Source: CAD feature listing. Evaluate the final solid. Frame: model axes, mm. Face numbers are marked on the shaded views. A direction names the side the tool comes from. Round coordinates to 2 decimals unless told otherwise and drop trailing zeros. Order: outer loops, then holes, each group sorted by start corner. A loop starts at its lowest first (then second) coordinate and runs counter-clockwise, first axis right, second up. Notation, with made-up numbers: (85.5, 7.25) -> (101.5, 7.25) arc R24 cw to (101.5, 25.25) -> close; hole circle Ø9 at (59.25, -34.75). An arc over 180 degrees is marked (long way). Answer as CSV lines item,"result".
from build123d import *

# Parameters (mm, degrees)
F0_W      = 165.1
F0_H      = 44.45
F1_DEPTH  = 22.86
F2_R      = 5.08
F3_DEPTH  = 5.334
F4_R      = 2.794
F5_DEPTH  = 25.4
F6_W      = 9.398
F6_H      = 16.51
F7_DEPTH  = 21.59
F8_W      = 2.286
F8_H      = 16.51
F9_DEPTH  = 8.128
F11_DEPTH = 25.4
F12_R     = 1.27
F13_DEPTH = 6.35


with BuildPart() as f1:
    # F0 (on Front) → F1 (new body)
    with BuildSketch(Plane.XZ):
        with Locations((22.303157, 29.753123)):
            Rectangle(F0_W, F0_H)
    extrude(amount=F1_DEPTH)

    # F2 (on face) → F3 (join)
    with BuildSketch(Plane(origin=(-60.246843, 0, 0), x_dir=(0, -1, 0), z_dir=(-1, 0, 0))):
        with Locations((9.652, 36.103123)):
            Circle(F2_R)
    extrude(amount=F3_DEPTH)

    # F4 (on face) → F5 (join)
    with BuildSketch(Plane(origin=(-65.580843, 0, 0), x_dir=(0, -1, 0), z_dir=(-1, 0, 0))):
        with Locations((9.652, 36.103123)):
            Circle(F4_R)
    extrude(amount=F5_DEPTH)

    # F6 (on face) → F7 (join)
    with BuildSketch(Plane.XZ.offset(22.86)):
        with Locations((-36.497843, 39.913123)):
            Rectangle(F6_W, F6_H)
        with Locations((-15.542843, 39.913123)):
            Rectangle(F6_W, F6_H)
        with Locations((5.412157, 39.913123)):
            Rectangle(F6_W, F6_H)
        with Locations((26.367157, 39.913123)):
            Rectangle(F6_W, F6_H)
        with Locations((47.322157, 39.913123)):
            Rectangle(F6_W, F6_H)
        with Locations((68.277157, 39.913123)):
            Rectangle(F6_W, F6_H)
        with Locations((89.232157, 39.913123)):
            Rectangle(F6_W, F6_H)
    extrude(amount=F7_DEPTH)

    # F8 (on face) → F9 (join)
    with BuildSketch(Plane.YZ.offset(104.853157)):
        with Locations((-1.143, 29.753123)):
            Rectangle(F8_W, F8_H)
    extrude(amount=F9_DEPTH)

    # F10 (on face) → F11 (cut)
    with BuildSketch(Plane.XZ.offset(2.286)):
        with BuildLine():
            Line((112.981157, 38.008123), (104.853157, 38.008123))
            Line((104.853157, 38.008123), (111.457157, 33.055123))
            ThreePointArc((111.457157, 33.055123), (112.578924, 31.711006), (112.981157, 30.007123))
            Line((112.981157, 30.007123), (112.981157, 31.912123))
            Line((112.981157, 31.912123), (112.981157, 38.008123))
        make_face()
        with BuildLine():
            Line((112.981157, 27.594123), (112.981157, 29.499123))
            ThreePointArc((112.981157, 29.499123), (112.578924, 27.795239), (111.457157, 26.451123))
            Line((111.457157, 26.451123), (104.853157, 21.498123))
            Line((104.853157, 21.498123), (112.981157, 21.498123))
            Line((112.981157, 21.498123), (112.981157, 27.594123))
        make_face()
        with BuildLine():
            Line((110.339557, 32.039123), (106.072357, 35.239523))
            ThreePointArc((106.072357, 35.239523), (105.27438, 35.311476), (104.853157, 34.629923))
            Line((104.853157, 34.629923), (104.853157, 29.753123))
            Line((104.853157, 29.753123), (111.355557, 29.753123))
            Line((111.355557, 29.753123), (111.355557, 30.007123))
            ThreePointArc((111.355557, 30.007123), (111.087402, 31.143045), (110.339557, 32.039123))
        make_face()
        with BuildLine():
            Line((111.355557, 29.753123), (104.853157, 29.753123))
            Line((104.853157, 29.753123), (104.853157, 24.876323))
            ThreePointArc((104.853157, 24.876323), (105.27438, 24.194769), (106.072357, 24.266723))
            Line((106.072357, 24.266723), (110.339557, 27.467123))
            ThreePointArc((110.339557, 27.467123), (111.087402, 28.3632), (111.355557, 29.499123))
            Line((111.355557, 29.499123), (111.355557, 29.753123))
        make_face()
    extrude(amount=-F11_DEPTH, mode=Mode.SUBTRACT)

    # F12 (on face) → F13 (cut)
    with BuildSketch(Plane(origin=(0, 0, 0), x_dir=(-1, 0, 0), z_dir=(0, 1, 0))):
        with Locations((47.546843, 29.753123)):
            Circle(F12_R)
    extrude(amount=-F13_DEPTH, mode=Mode.SUBTRACT)


solid = f1.part
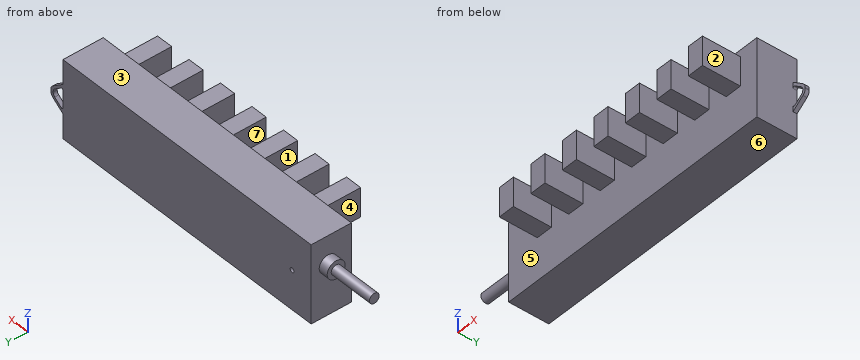
1. Section query A-A on y = -27.5. Return loops of the section in (x, z), and give its area (3 significant figures).
Results below:
outline,"(-41.2, 31.66) -> (-31.8, 31.66) -> (-31.8, 48.17) -> (-41.2, 48.17) -> close; (-20.24, 31.66) -> (-10.84, 31.66) -> (-10.84, 48.17) -> (-20.24, 48.17) -> close; (0.71, 31.66) -> (10.11, 31.66) -> (10.11, 48.17) -> (0.71, 48.17) -> close; (21.67, 31.66) -> (31.07, 31.66) -> (31.07, 48.17) -> (21.67, 48.17) -> close; (42.62, 31.66) -> (52.02, 31.66) -> (52.02, 48.17) -> (42.62, 48.17) -> close; (63.58, 31.66) -> (72.98, 31.66) -> (72.98, 48.17) -> (63.58, 48.17) -> close; (84.53, 31.66) -> (93.93, 31.66) -> (93.93, 48.17) -> (84.53, 48.17) -> close"
area,"1,090 mm2"
2. Line query: L1, parallel to Y at x = 18.5, z = 33.5; L2, parallel to X at y = -22.5, z = 36.5; L3, parallel to Z at x = -11.5, y = -26. Output: solid intervals per line, ascending. Write a range as [from, to].
Results below:
L1,"[-22.86, 0]"
L2,"[-60.25, 104.85]"
L3,"[31.66, 48.17]"
3. Reachability of the marked faces 1, 2 and 3 from +Z, -Z, +X, -X, +Y, -Y: full face, straight path, thin tool, end or side. Return the list, or none.
Results below:
face 1,"+Z, -Z, -Y"
face 2,"+Z, -Z, +X, -Y"
face 3,"+Z, +X, -X, +Y, -Y"
4. Pin query (flat end, axial travel): pin 1 (18 mm diameter, centred on y = -31.5, z = 41.5, fed in from -X); pin 2 (8.5 mm diameter, centred on y = -38, z = 40, fed in from -X); pin 3 (10.5 mm diameter, centred on x = 91, y = -35.5, fed in from +Z). Return the tip coordinate at first contact, or that it passes through.
Results below:
pin 1,"x = -60.25"
pin 2,"x = -41.2"
pin 3,"z = 48.17"
5. Section query C-C on z = 19. Return loops of the section in (x, y).
Results below:
outline,"(-60.25, -22.86) -> (104.85, -22.86) -> (104.85, 0) -> (-60.25, 0) -> close"
6. Mould query, pull axis X, two halves, no side actions, for the marked faces 4, 5, 6 and 7. Classes: released by +X, released by -X, zero draft, split by the parting line, or undercut.
Results below:
face 4,"released by -X"
face 5,"undercut"
face 6,"zero draft"
face 7,"undercut"
7. Section query D-D on x = 34. Return loops of the section in (y, z).
Results below:
outline,"(-22.86, 7.53) -> (0, 7.53) -> (0, 51.98) -> (-22.86, 51.98) -> close"
8. Section query B-B on x = 87. Return loops of the section in (y, z).
Results below:
outline,"(-44.45, 31.66) -> (-22.86, 31.66) -> (-22.86, 7.53) -> (0, 7.53) -> (0, 51.98) -> (-22.86, 51.98) -> (-22.86, 48.17) -> (-44.45, 48.17) -> close"
